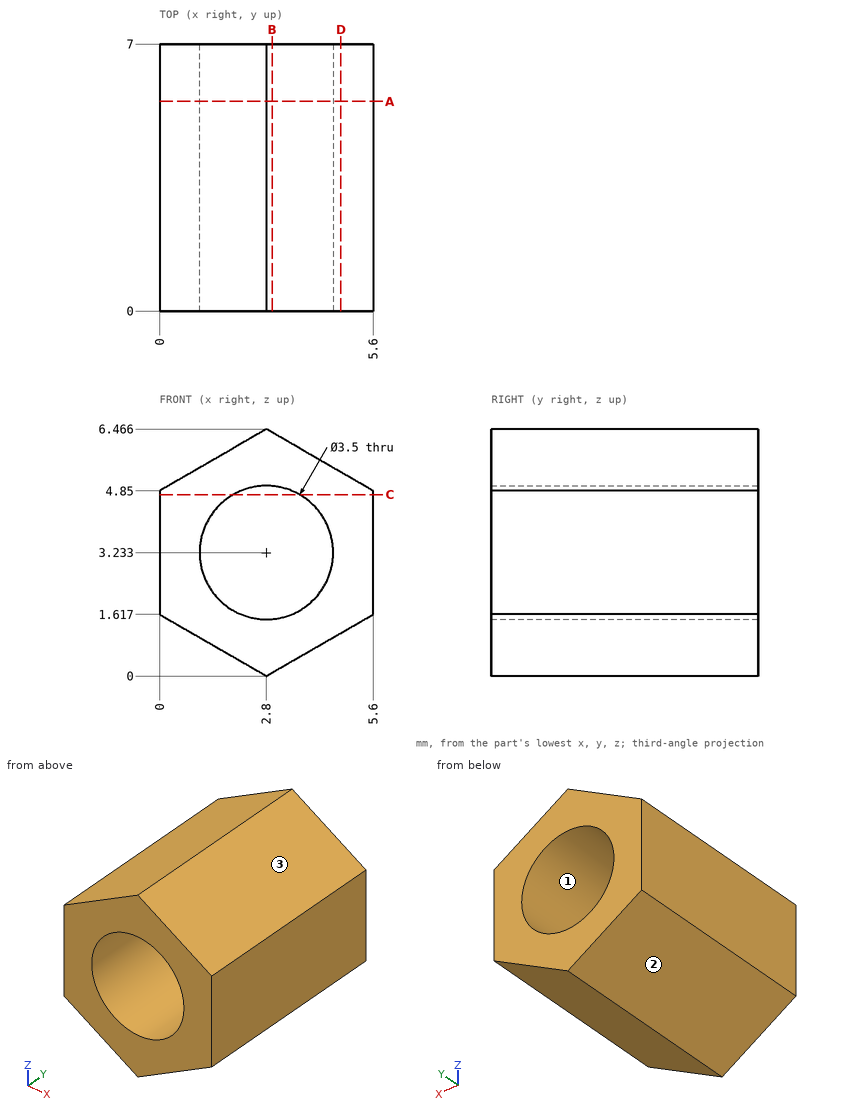
Print and shaded views of the part. All mm, measured from the part's lowest x, y and z. Round coordinates to 2 decimals unless told otherwise and drop trailing zeros. Write each loop counter-clockwise with the first axis right and the second up, starting at its lowest first coordinate (ties: lowest second). Pieces come first, ordered by that corner, then holes.
(1) Mould opens along Z. For the marked faces 1, 2 and 3 say: pulls with the +Z half, pulls with the -Z half, needs draft (parallel to the pull), parting line crosses it, or undercut.
(2) Slice it at D-D, the plane x = 4.75. Write the cut outline in (y, z) (1 decimal).
(3) Probe line 1 along X through (y, z) = (5, 4.25) (1 decimal); line 2 along Z through (x, y) = (3.1, 2.5) (1 decimal); line 3 along X through (y, z) = (2.25, 4.5) (1 decimal). List the from-to ranges inside material, lowest first.
(4) Slice it at B-B, the plane x = 2.95. Write the cut outline in (y, z).
(5) Slice it at C-C, the plane z = 4.75. Write the cut outline in (x, y), and give its area (3 significant figures).
(6) Drop flat-ended pins along their axis: P1, Ø1, axis at x = 4, y = 5.5, coming from the -Z side (1 decimal); P2, Ø3, axis at x = 2.8, z = 3.23, coming from the -Y side. Give the stop position or say it passes through.
(7) Slice it at A-A, the plane y = 5.5. Write the cut outline in (x, z).
From the geometry:
1. face 1: undercut
1. face 2: pulls with the -Z half
1. face 3: pulls with the +Z half
2. outline: (0, 1.1) - (7, 1.1) - (7, 5.3) - (0, 5.3) - close
3. line 1: x = 0 to 1.4, 4.2 to 5.6
3. line 2: z = 0.2 to 1.5, 5 to 6.3
3. line 3: x = 0 to 1.6, 4 to 5.6
4. outline: (0, 0.09) - (7, 0.09) - (7, 1.49) - (0, 1.49) - close; (0, 4.98) - (7, 4.98) - (7, 6.38) - (0, 6.38) - close
5. outline: (0, 0) - (1.93, 0) - (1.93, 7) - (0, 7) - close; (3.67, 0) - (5.6, 0) - (5.6, 7) - (3.67, 7) - close
5. area: 27.0 mm2
6. P1: stops at z = 0.4
6. P2: passes through
7. outline: (0, 1.62) - (2.8, 0) - (5.6, 1.62) - (5.6, 4.85) - (2.8, 6.47) - (0, 4.85) - close; hole circle Ø3.5 at (2.8, 3.23)
